Model file for the job. Use its own axes, mm. A direction names the side the tool comes from. Coordinates: 2 decimals unless noted, no trailing zeros. Write each loop counter-clockwise with the first axis right and the second up, starting at its lowest first coordinate (ties: lowest second). Pieces come first, ordered by that corner, then holes. Notation, with made-up numbers: (-20.75, 40.5) - (10.25, 40.5) arc R19 ccw to (10.25, 53.5) - close; hole circle Ø7 at (34, 7.5). An arc over 180 degrees is marked (long way). Put each result on its own line as item: value. Start each with the question number.
1. Drop flat-ended pins along their axis: P1, Ø3, axis at y = -5.5, z = 16, coming from the +X side; P2, Ø6, axis at y = 9.5, z = 15, coming from the +X side; P3, Ø1.5, axis at x = -57.5, z = 2.5, coming from the -Y side. Give the stop position or say it passes through.
2. Saw through at B-B, the plane x = -36. Write the cut outline in (y, z), plus the area to 3 significant figures.
3. Saw through at A-A, the plane y = -11. Write the cut outline in (x, z).
4. Which spindle directions (+Z, -Z, +X, -X, +Y, -Y) get a long thin tool onto all of the face, cutting with end or side? Do faces 5 (the face through (-21.388, 53, 9)), 6 (the face through (-57.902, 51.402, 9.392)), 7 (the face through (-29.82, -11.73, 9.39)), 8 (the face through (5.49, -3.27, 9.39)). Say none if no direction does.
5. Saw through at C-C, the plane y = 59. Write the cut outline in (x, z).
6. Pull direction X, two halves, no side cores. Call faces 1 (the face through (3.789, -26.094, 9.392)), 2 (the face through (-23.575, 23.095, 9.392)), 3 (the face through (-18.168, 70.494, 9.392)), 4 (the face through (-67.75, 8.43, 9.39)): released by +X, released by -X, zero draft, split by the parting line, or undercut.
7. Saw through at D-D, the plane x = 13. Write the cut outline in (y, z), plus the area to 3 significant figures.
8. Drill centre lines: L1, parallel to Y at x = -34.5, z = 4; L2, parallel to Y at x = 14, z = 8.75; L3, parallel to X at y = 52.5, z = 16.5. Where is each one in solid material? Low to high. Write a range as from..to.
```python
from build123d import *

# Parameters (mm, degrees)
BOSS_EXTRUDE1_DEPTH = 19.05


with BuildPart() as part:
    # Sketch1 → Boss-Extrude1 (new body)
    with BuildSketch(Plane.XY):
        with BuildLine():
            Line((-68.348679847, 27.880791406), (-34.028682265, 20.047475917))
            ThreePointArc((-34.028682265, 20.047475917), (-32.480984204, 19.694223934), (-34.028682265, 19.340971952))
            Line((-34.028682265, 19.340971952), (-68.348679847, 11.507656462))
            ThreePointArc((-68.348679847, 11.507656462), (-67.739001659, 8.390160489), (-66.935671916, 5.31686422))
            Line((-66.935671916, 5.31686422), (-32.615674334, 13.150179709))
            ThreePointArc((-32.615674334, 13.150179709), (-31.067976273, 13.503431692), (-32.309133752, 12.513641632))
            Line((-32.309133752, 12.513641632), (-59.831634906, -9.434820634))
            ThreePointArc((-59.831634906, -9.434820634), (-57.92970303, -11.979058), (-55.872474664, -14.399450548))
            Line((-55.872474664, -14.399450548), (-28.34997351, 7.549011718))
            ThreePointArc((-28.34997351, 7.549011718), (-27.108816032, 8.538801778), (-27.797606467, 7.1085137))
            Line((-27.797606467, 7.1085137), (-43.071442298, -24.60793321))
            ThreePointArc((-43.071442298, -24.60793321), (-40.253957668, -26.074994555), (-37.350289987, -27.363094953))
            Line((-37.350289987, -27.363094953), (-22.076454156, 4.353351957))
            ThreePointArc((-22.076454156, 4.353351957), (-21.38766372, 5.783640035), (-21.38766372, 4.196140035))
            Line((-21.38766372, 4.196140035), (-21.38766372, -31.006460233))
            ThreePointArc((-21.38766372, -31.006460233), (-18.21266372, -31.105776066), (-15.03766372, -31.006460233))
            Line((-15.03766372, -31.006460233), (-15.03766372, 4.196140035))
            ThreePointArc((-15.03766372, 4.196140035), (-15.03766372, 5.783640035), (-14.348873285, 4.353351957))
            Line((-14.348873285, 4.353351957), (0.924962546, -27.363094953))
            ThreePointArc((0.924962546, -27.363094953), (3.828630227, -26.074994555), (6.646114857, -24.60793321))
            Line((6.646114857, -24.60793321), (-8.627720973, 7.1085137))
            ThreePointArc((-8.627720973, 7.1085137), (-9.316511409, 8.538801778), (-8.075353931, 7.549011718))
            Line((-8.075353931, 7.549011718), (19.447147223, -14.399450548))
            ThreePointArc((19.447147223, -14.399450548), (21.504375589, -11.979058), (23.406307465, -9.434820634))
            Line((23.406307465, -9.434820634), (-4.116193689, 12.513641632))
            ThreePointArc((-4.116193689, 12.513641632), (-5.357351167, 13.503431692), (-3.809653107, 13.150179709))
            Line((-3.809653107, 13.150179709), (30.510344475, 5.31686422))
            ThreePointArc((30.510344475, 5.31686422), (31.313674218, 8.390160489), (31.923352406, 11.507656462))
            Line((31.923352406, 11.507656462), (-2.396645176, 19.340971952))
            ThreePointArc((-2.396645176, 19.340971952), (-3.944343237, 19.694223934), (-2.396645176, 20.047475917))
            Line((-2.396645176, 20.047475917), (31.923352406, 27.880791406))
            ThreePointArc((31.923352406, 27.880791406), (31.313674218, 30.998287379), (30.510344475, 34.071583649))
            Line((30.510344475, 34.071583649), (-3.809653107, 26.238268159))
            ThreePointArc((-3.809653107, 26.238268159), (-5.357351167, 25.885016177), (-4.116193689, 26.874806237))
            Line((-4.116193689, 26.874806237), (23.406307465, 48.823268503))
            ThreePointArc((23.406307465, 48.823268503), (21.504375589, 51.367505869), (19.447147223, 53.787898417))
            Line((19.447147223, 53.787898417), (-8.075353931, 31.839436151))
            ThreePointArc((-8.075353931, 31.839436151), (-9.316511409, 30.84964609), (-8.627720973, 32.279934168))
            Line((-8.627720973, 32.279934168), (6.646114857, 63.996381078))
            ThreePointArc((6.646114857, 63.996381078), (3.828630227, 65.463442424), (0.924962546, 66.751542822))
            Line((0.924962546, 66.751542822), (-14.348873285, 35.035095912))
            ThreePointArc((-14.348873285, 35.035095912), (-15.03766372, 33.604807834), (-15.03766372, 35.192307834))
            Line((-15.03766372, 35.192307834), (-15.03766372, 70.394908101))
            ThreePointArc((-15.03766372, 70.394908101), (-18.21266372, 70.494223934), (-21.38766372, 70.394908101))
            Line((-21.38766372, 70.394908101), (-21.38766372, 35.192307834))
            ThreePointArc((-21.38766372, 35.192307834), (-21.38766372, 33.604807834), (-22.076454156, 35.035095912))
            Line((-22.076454156, 35.035095912), (-37.350289987, 66.751542822))
            ThreePointArc((-37.350289987, 66.751542822), (-40.253957668, 65.463442424), (-43.071442298, 63.996381078))
            Line((-43.071442298, 63.996381078), (-27.797606467, 32.279934168))
            ThreePointArc((-27.797606467, 32.279934168), (-27.108816032, 30.84964609), (-28.34997351, 31.839436151))
            Line((-28.34997351, 31.839436151), (-55.872474664, 53.787898417))
            ThreePointArc((-55.872474664, 53.787898417), (-57.92970303, 51.367505869), (-59.831634906, 48.823268503))
            Line((-59.831634906, 48.823268503), (-32.309133752, 26.874806237))
            ThreePointArc((-32.309133752, 26.874806237), (-31.067976273, 25.885016177), (-32.615674334, 26.238268159))
            Line((-32.615674334, 26.238268159), (-66.935671916, 34.071583649))
            ThreePointArc((-66.935671916, 34.071583649), (-67.739001659, 30.998287379), (-68.348679847, 27.880791406))
        make_face()
        Polygon((-10.889375563, 19.329828678), (-14.866595191, 13.169872723), (-22.189883348, 13.534267979), (-25.535951877, 20.05861919), (-21.55873225, 26.218575146), (-14.235444093, 25.854179889), align=None, mode=Mode.SUBTRACT)
    extrude(amount=BOSS_EXTRUDE1_DEPTH)


solid = part.part
```
Final values:
1. P1: stops at x = 20.35
1. P2: stops at x = 31.92
1. P3: stops at y = -13.4
2. outline: (-24.56, 0) - (-9.92, 0) - (-9.92, 19.05) - (-24.56, 19.05) - close; (1.45, 0) - (9.57, 0) - (9.57, 19.05) - (1.45, 19.05) - close; (12.38, 0) - (18.89, 0) - (18.89, 19.05) - (12.38, 19.05) - close; (20.5, 0) - (27.01, 0) - (27.01, 19.05) - (20.5, 19.05) - close; (29.82, 0) - (37.94, 0) - (37.94, 19.05) - (29.82, 19.05) - close; (49.31, 0) - (63.95, 0) - (63.95, 19.05) - (49.31, 19.05) - close
2. area: 1,120 mm²
3. outline: (-58.69, 0) - (-51.61, 0) - (-51.61, 19.05) - (-58.69, 19.05) - close; (-36.52, 0) - (-29.47, 0) - (-29.47, 19.05) - (-36.52, 19.05) - close; (-21.39, 0) - (-15.04, 0) - (-15.04, 19.05) - (-21.39, 19.05) - close; (-6.96, 0) - (0.09, 0) - (0.09, 19.05) - (-6.96, 19.05) - close; (15.18, 0) - (22.27, 0) - (22.27, 19.05) - (15.18, 19.05) - close
4. face 5: +Z, -Z, +Y
4. face 6: +Z, -Z, -X, +Y
4. face 7: +Z, -Z, -Y
4. face 8: +Z, -Z
5. outline: (-40.67, 0) - (-33.62, 0) - (-33.62, 19.05) - (-40.67, 19.05) - close; (-21.39, 0) - (-15.04, 0) - (-15.04, 19.05) - (-21.39, 19.05) - close; (-2.81, 0) - (4.24, 0) - (4.24, 19.05) - (-2.81, 19.05) - close
6. face 1: released by +X
6. face 2: undercut
6. face 3: split by the parting line
6. face 4: released by -X
7. outline: (-9.26, 0) - (-1.14, 0) - (-1.14, 19.05) - (-9.26, 19.05) - close; (9.31, 0) - (15.83, 0) - (15.83, 19.05) - (9.31, 19.05) - close; (23.56, 0) - (30.07, 0) - (30.07, 19.05) - (23.56, 19.05) - close; (40.52, 0) - (48.65, 0) - (48.65, 19.05) - (40.52, 19.05) - close
7. area: 558 mm²
8. L1: y = -21.44..-6.81, 2.64..10.77, 12.72..19.23, 20.16..26.67, 28.62..36.74, 46.2..60.83
8. L2: y = -10.06..-1.93, 9.09..15.6, 23.79..30.3, 41.32..49.44
8. L3: x = -57..-54.26, -37.54..-30.49, -21.39..-15.04, -5.94..1.11, 17.83..20.57
